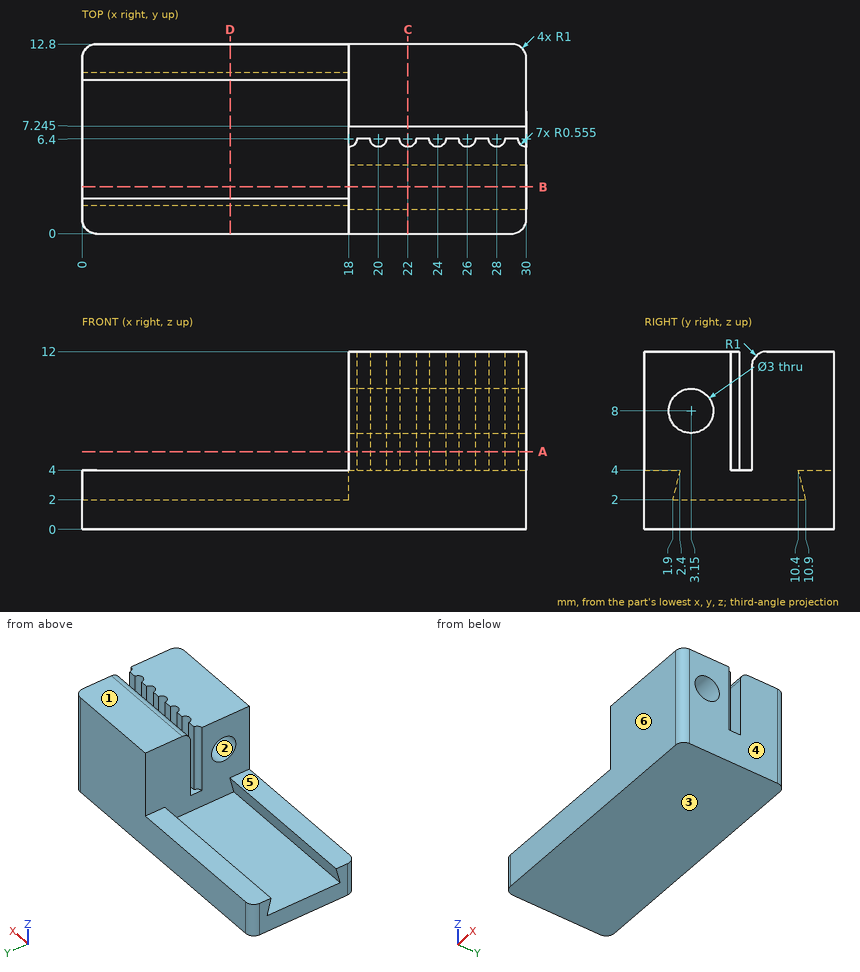
Here's the drawing with two shaded views (mm, measured from the low corner). I have some questions. A direction names the side the tool comes from. Give positions to 0.01 mm unless a question says otherwise; leave off trailing zeros. Loops run counter-clockwise (first coordinate to the right, second up) from the corner with the lowest first, then second, coordinate; pieces in that order, holes last. Notation, with made-up numbers: (67, 78) - (94, 78) arc R16 ccw to (94, 89) - close; hole circle Ø3 at (1, 66.25). An arc over 180 degrees is marked (long way). One line per item, written item: value.
(1) If we section it at A-A, the plane z = 5.25: List the corners of the cut face in (x, y) for me (3 decimals), plus the area to 3 significant figures.
Verdict:
outline: (18, 0) - (29, 0) arc R1 ccw to (30, 1) - (30, 5.845) arc R0.555 cw to (29.445, 6.4) - (28.555, 6.4) arc R0.555 cw to (27.445, 6.4) - (26.555, 6.4) arc R0.555 cw to (25.445, 6.4) - (24.555, 6.4) arc R0.555 cw to (23.445, 6.4) - (22.555, 6.4) arc R0.555 cw to (21.445, 6.4) - (20.555, 6.4) arc R0.555 cw to (19.445, 6.4) - (18.555, 6.4) arc R0.555 cw to (18, 5.845) - close; (18, 7.245) - (30, 7.245) - (30, 11.8) arc R1 ccw to (29, 12.8) - (18, 12.8) - close
area: 140 mm^2
(2) If we mould it in two halves opening along Z, with no side actions, what happens to the marked faces 1, 2, 3 and 4? For each: released by +Z, released by -Z, zero draft, split by the parting line, or undercut.
Verdict:
face 1: released by +Z
face 2: undercut
face 3: released by -Z
face 4: zero draft
(3) I'm going to push flat-ended pins straight in: pin 1 (0.7 mm diameter, centred on x = 5.5, y = 1.5, fed in from +Z); pin 2 (5 mm diameter, centred on y = 4.5, z = 8.5, fed in from -X); pin 3 (1 mm diameter, centred on x = 6, y = 8, fed in from +Z). Where does each tip first touch, or does it pass through?
Verdict:
pin 1: z = 4
pin 2: x = 18
pin 3: z = 2
(4) If we section it at B-B, the plane y = 3.15: List the corners of the cut face in (x, z) for me, plus the area to 3 significant figures.
Verdict:
outline: (0, 0) - (30, 0) - (30, 6.5) - (18, 6.5) - (18, 2) - (0, 2) - close; (18, 9.5) - (30, 9.5) - (30, 12) - (18, 12) - close
area: 144 mm^2
(5) I need wall thicknesses on line 1 along Y through (x, z) = (26, 8) (3 decimals); line 2 along Y through (x, z) = (23, 8) (3 decimals); line 3 along Y through (x, z) = (25, 11) (3 decimals). Which ranges of each line are inside material? Lowest first, please.
Verdict:
line 1: 0 to 1.65, 4.65 to 5.845, 7.245 to 12.8
line 2: 0 to 1.65, 4.65 to 6.4, 7.245 to 12.8
line 3: 0 to 6.4, 7.245 to 12.8
(6) If we section it at D-D, the plane x = 10: List the corners of the cut face in (y, z) for me.
Verdict:
outline: (0, 0) - (12.8, 0) - (12.8, 4) - (10.4, 4) - (10.9, 2) - (1.9, 2) - (2.4, 4) - (0, 4) - close
(7) If we section it at C-C, the plane x = 22: List the corners of the cut face in (y, z) for me (3 decimals), plus the area to 3 significant figures.
Verdict:
outline: (0, 0) - (12.8, 0) - (12.8, 12) - (8.245, 12) arc R1 ccw to (7.245, 11) - (7.245, 4) - (5.845, 4) - (5.845, 12) - (0, 12) - close; hole circle Ø3 at (3.15, 8)
area: 135 mm^2
(8) On a 3-axis mill with a long thin cutter (end or side, diameter ignored), from which of +Z, -Z, +X, -X, +Y, -Y can I reach the whole of each face in a straight line? I mean the marked faces 5 and 6. Say none if no direction works.
Verdict:
face 5: +Z, -X, +Y, -Y
face 6: +Z, -Z, +X, -X, -Y
